from build123d import *

# Parameters (mm, degrees)
SKETCH1_W                 = 62.1
SKETCH1_H                 = 0.7
BASE_FLANGE1_DEPTH        = 87.8
EDGE_FLANGE1_DEPTH        = 87.8
EDGE_FLANGE2_DEPTH        = 87.8
EDGE_FLANGE3_DEPTH        = 62.1
CUT_EXTRUDE2_DEPTH        = 0.7
SKETCH14_R                = 1.7
CUT_EXTRUDE3_DEPTH        = 0.7
EDGE_FLANGE4_DEPTH        = 19
EDGE_FLANGE5_DEPTH        = 19
EDGE_FLANGE6_DEPTH        = 62.1
EDGE_FLANGE7_DEPTH        = 19
EDGE_FLANGE8_DEPTH        = 19
SKETCH32_W                = 10.5
SKETCH32_H                = 8
CUT_EXTRUDE5_DEPTH        = 0.7
FLAT_PATTERN1_START       = -20.7
FLAT_PATTERN1_OUTLINE_R   = 1.7
FLAT_PATTERN1_DEPTH       = 20
FLAT_PATTERN1_START_2     = -0.7
FLAT_PATTERN1_2_OUTLINE_R = 1.7
FLAT_PATTERN1_2_DEPTH     = 0.7


with BuildPart() as part:
    # Base-Flange1: sheet metal written as solids
    # Sketch1 → Base-Flange1 (new body)
    with BuildSketch(Plane.XY):
        with Locations((31.05, -0.35)):
            Rectangle(SKETCH1_W, SKETCH1_H)
    extrude(amount=BASE_FLANGE1_DEPTH)

    # Edge-Flange1: sheet metal written as solids
    # Edge-Flange1 section (on a plane across the edge) → Edge-Flange1 (add)
    with BuildSketch(Plane(origin=(63.1, -0.7, 0), x_dir=(-1, 0, 0), z_dir=(0, 0, 1))):
        with BuildLine():
            Line((-0.7, 1), (-0.7, 20))
            Line((-0.7, 20), (0, 20))
            Line((0, 20), (0, 1))
            ThreePointArc((0, 1), (0.292893219, 0.292893219), (1, 0))
            Line((1, 0), (1, -0.7))
            ThreePointArc((1, -0.7), (-0.202081528, -0.202081528), (-0.7, 1))
        make_face()
    extrude(amount=EDGE_FLANGE1_DEPTH)

    # Edge-Flange2: sheet metal written as solids
    # Edge-Flange2 section (on a plane across the edge) → Edge-Flange2 (add)
    with BuildSketch(Plane(origin=(-1, -0.7, 87.8), x_dir=(1, 0, 0), z_dir=(0, 0, -1))):
        with BuildLine():
            Line((-0.7, 1), (-0.7, 20))
            Line((-0.7, 20), (0, 20))
            Line((0, 20), (0, 1))
            ThreePointArc((0, 1), (0.292893219, 0.292893219), (1, 0))
            Line((1, 0), (1, -0.7))
            ThreePointArc((1, -0.7), (-0.202081528, -0.202081528), (-0.7, 1))
        make_face()
    extrude(amount=EDGE_FLANGE2_DEPTH)

    # Edge-Flange3: sheet metal written as solids
    # Edge-Flange3 section (on a plane across the edge) → Edge-Flange3 (add)
    with BuildSketch(Plane(origin=(62.1, -0.7, 88.8), x_dir=(0, 0, -1), z_dir=(-1, 0, 0))):
        with BuildLine():
            Line((-0.7, 1), (-0.7, 20))
            Line((-0.7, 20), (0, 20))
            Line((0, 20), (0, 1))
            ThreePointArc((0, 1), (0.292893219, 0.292893219), (1, 0))
            Line((1, 0), (1, -0.7))
            ThreePointArc((1, -0.7), (-0.202081528, -0.202081528), (-0.7, 1))
        make_face()
    extrude(amount=EDGE_FLANGE3_DEPTH)

    # Sketch13 → Cut-Extrude2 (cut)
    with BuildSketch(Plane.XY.offset(89.5)):
        with BuildLine():
            Line((38.05, -13.35), (38.05, -20.7))
            Line((38.05, -20.7), (48.05, -20.7))
            Line((48.05, -20.7), (48.05, -13.35))
            ThreePointArc((48.05, -13.35), (43.05, -8.35), (38.05, -13.35))
        make_face()
    extrude(amount=-CUT_EXTRUDE2_DEPTH, mode=Mode.SUBTRACT)

    # Sketch14 → Cut-Extrude3 (cut)
    with BuildSketch(Plane(origin=(0, 0, 0), x_dir=(1, 0, 0), z_dir=(0, 1, 0))):
        with Locations(Location((6.55, -7.2, 0), (0, 0, 270))):
            Circle(SKETCH14_R)
        with Locations(Location((55.55, -7.2, 0), (0, 0, 270))):
            Circle(SKETCH14_R)
        with Locations(Location((8.05, -80.7, 0), (0, 0, 270))):
            Circle(SKETCH14_R)
        with Locations(Location((54.05, -80.7, 0), (0, 0, 270))):
            Circle(SKETCH14_R)
    extrude(amount=-CUT_EXTRUDE3_DEPTH, mode=Mode.SUBTRACT)

    # Edge-Flange4: sheet metal written as solids
    # Edge-Flange4 section (on a plane across the edge) → Edge-Flange4 (add)
    with BuildSketch(Plane(origin=(64.1, -1.7, 88.8), x_dir=(-1, 0, 0), z_dir=(0, -1, 0))):
        with BuildLine():
            Line((-0.7, 2), (-0.7, 20))
            Line((-0.7, 20), (0, 20))
            Line((0, 20), (0, 2))
            ThreePointArc((0, 2), (0.585786438, 0.585786438), (2, 0))
            Line((2, 0), (2, -0.7))
            ThreePointArc((2, -0.7), (0.090811691, 0.090811691), (-0.7, 2))
        make_face()
    extrude(amount=EDGE_FLANGE4_DEPTH)

    # Edge-Flange5: sheet metal written as solids
    # Edge-Flange5 section (on a plane across the edge) → Edge-Flange5 (add)
    with BuildSketch(Plane(origin=(-2, -20.7, 88.8), x_dir=(1, 0, 0), z_dir=(0, 1, 0))):
        with BuildLine():
            Line((-0.7, 2), (-0.7, 20))
            Line((-0.7, 20), (0, 20))
            Line((0, 20), (0, 2))
            ThreePointArc((0, 2), (0.585786438, 0.585786438), (2, 0))
            Line((2, 0), (2, -0.7))
            ThreePointArc((2, -0.7), (0.090811691, 0.090811691), (-0.7, 2))
        make_face()
    extrude(amount=EDGE_FLANGE5_DEPTH)

    # Edge-Flange6: sheet metal written as solids
    # Edge-Flange6 section (on a plane across the edge) → Edge-Flange6 (add)
    with BuildSketch(Plane(origin=(0, -0.7, -1), x_dir=(0, 0, 1), z_dir=(1, 0, 0))):
        with BuildLine():
            Line((-0.7, 1), (-0.7, 20))
            Line((-0.7, 20), (0, 20))
            Line((0, 20), (0, 1))
            ThreePointArc((0, 1), (0.292893219, 0.292893219), (1, 0))
            Line((1, 0), (1, -0.7))
            ThreePointArc((1, -0.7), (-0.202081528, -0.202081528), (-0.7, 1))
        make_face()
    extrude(amount=EDGE_FLANGE6_DEPTH)

    # Edge-Flange7: sheet metal written as solids
    # Edge-Flange7 section (on a plane across the edge) → Edge-Flange7 (add)
    with BuildSketch(Plane(origin=(64.1, -20.7, -1), x_dir=(-1, 0, 0), z_dir=(0, 1, 0))):
        with BuildLine():
            Line((-0.7, 2), (-0.7, 20))
            Line((-0.7, 20), (0, 20))
            Line((0, 20), (0, 2))
            ThreePointArc((0, 2), (0.585786438, 0.585786438), (2, 0))
            Line((2, 0), (2, -0.7))
            ThreePointArc((2, -0.7), (0.090811691, 0.090811691), (-0.7, 2))
        make_face()
    extrude(amount=EDGE_FLANGE7_DEPTH)

    # Edge-Flange8: sheet metal written as solids
    # Edge-Flange8 section (on a plane across the edge) → Edge-Flange8 (add)
    with BuildSketch(Plane(origin=(-2, -1.7, -1), x_dir=(1, 0, 0), z_dir=(0, -1, 0))):
        with BuildLine():
            Line((-0.7, 2), (-0.7, 20))
            Line((-0.7, 20), (0, 20))
            Line((0, 20), (0, 2))
            ThreePointArc((0, 2), (0.585786438, 0.585786438), (2, 0))
            Line((2, 0), (2, -0.7))
            ThreePointArc((2, -0.7), (0.090811691, 0.090811691), (-0.7, 2))
        make_face()
    extrude(amount=EDGE_FLANGE8_DEPTH)

    # Sketch32 → Cut-Extrude5 (cut)
    with BuildSketch(Plane(origin=(0, 0, -1.7), x_dir=(-1, 0, 0), z_dir=(0, 0, -1))):
        with Locations((-49.8006007, -16.7)):
            Rectangle(SKETCH32_W, SKETCH32_H)
    extrude(amount=-CUT_EXTRUDE5_DEPTH, mode=Mode.SUBTRACT)

    # Flat-Pattern1: read off the stored shape, not the designer's step
    # Flat-Pattern1 outline → Flat-Pattern1 (cut)
    with BuildSketch(Plane(origin=(0, 0, 0), x_dir=(1, 0, 0), z_dir=(0, 1, 0)).offset(FLAT_PATTERN1_START)):
        with BuildLine():
            Line((-1.7, 0), (-1.7, -87.8))
            Line((-1.7, -87.8), (0, -87.8))
            Line((0, -87.8), (0, -88.5))
            Line((0, -88.5), (-1.053565375, -88.5))
            ThreePointArc((-1.053565375, -88.5), (-1.747445385, -87.772848716), (-2, -86.8))
            Line((-2, -86.8), (-2, -68.8))
            Line((-2, -68.8), (-2.7, -68.8))
            Line((-2.7, -68.8), (-2.7, -86.8))
            ThreePointArc((-2.7, -86.8), (-2.54495263, -87.701784958), (-2.097617696, -88.5))
            Line((-2.097617696, -88.5), (-18.7, -88.5))
            Line((-18.7, -88.5), (-18.7, -107.5))
            Line((-18.7, -107.5), (38.05, -107.5))
            Line((38.05, -107.5), (38.05, -100.15))
            ThreePointArc((38.05, -100.15), (43.05, -95.15), (48.05, -100.15))
            Line((48.05, -100.15), (48.05, -107.5))
            Line((48.05, -107.5), (80.8, -107.5))
            Line((80.8, -107.5), (80.8, -88.5))
            Line((80.8, -88.5), (64.197617696, -88.5))
            ThreePointArc((64.197617696, -88.5), (64.64495263, -87.701784958), (64.8, -86.8))
            Line((64.8, -86.8), (64.8, -68.8))
            Line((64.8, -68.8), (64.1, -68.8))
            Line((64.1, -68.8), (64.1, -86.8))
            ThreePointArc((64.1, -86.8), (63.847445385, -87.772848716), (63.153565375, -88.5))
            Line((63.153565375, -88.5), (62.1, -88.5))
            Line((62.1, -88.5), (62.1, -87.8))
            Line((62.1, -87.8), (63.8, -87.8))
            Line((63.8, -87.8), (63.8, 0))
            Line((63.8, 0), (62.1, 0))
            Line((62.1, 0), (62.1, 0.7))
            Line((62.1, 0.7), (63.153565375, 0.7))
            ThreePointArc((63.153565375, 0.7), (63.847445385, -0.027151284), (64.1, -1))
            Line((64.1, -1), (64.1, -19))
            Line((64.1, -19), (64.8, -19))
            Line((64.8, -19), (64.8, -1))
            ThreePointArc((64.8, -1), (64.009188309, 0.909188309), (62.1, 1.7))
            Line((62.1, 1.7), (0, 1.7))
            ThreePointArc((0, 1.7), (-1.909188309, 0.909188309), (-2.7, -1))
            Line((-2.7, -1), (-2.7, -19))
            Line((-2.7, -19), (-2, -19))
            Line((-2, -19), (-2, -1))
            ThreePointArc((-2, -1), (-1.747445385, -0.027151284), (-1.053565375, 0.7))
            Line((-1.053565375, 0.7), (0, 0.7))
            Line((0, 0.7), (0, 0))
            Line((0, 0), (-1.7, 0))
        make_face()
        with Locations((55.55, -7.2)):
            Circle(FLAT_PATTERN1_OUTLINE_R, mode=Mode.SUBTRACT)
        with Locations((8.05, -80.7)):
            Circle(FLAT_PATTERN1_OUTLINE_R, mode=Mode.SUBTRACT)
        with Locations((54.05, -80.7)):
            Circle(FLAT_PATTERN1_OUTLINE_R, mode=Mode.SUBTRACT)
        with Locations((6.55, -7.2)):
            Circle(FLAT_PATTERN1_OUTLINE_R, mode=Mode.SUBTRACT)
    extrude(amount=FLAT_PATTERN1_DEPTH, mode=Mode.SUBTRACT)

    # Flat-Pattern1 2 outline → Flat-Pattern1 2 (add)
    with BuildSketch(Plane(origin=(0, 0, 0), x_dir=(1, 0, 0), z_dir=(0, 1, 0)).offset(FLAT_PATTERN1_START_2)):
        with BuildLine():
            Line((0, -87.8), (0, -88.5))
            Line((0, -88.5), (-18.7, -88.5))
            Line((-18.7, -88.5), (-18.7, -107.5))
            Line((-18.7, -107.5), (38.05, -107.5))
            Line((38.05, -107.5), (38.05, -100.15))
            ThreePointArc((38.05, -100.15), (43.05, -95.15), (48.05, -100.15))
            Line((48.05, -100.15), (48.05, -107.5))
            Line((48.05, -107.5), (80.8, -107.5))
            Line((80.8, -107.5), (80.8, -88.5))
            Line((80.8, -88.5), (62.1, -88.5))
            Line((62.1, -88.5), (62.1, -87.8))
            Line((62.1, -87.8), (81.8, -87.8))
            Line((81.8, -87.8), (81.8, 0))
            Line((81.8, 0), (62.1, 0))
            Line((62.1, 0), (62.1, 0.7))
            Line((62.1, 0.7), (80.8, 0.7))
            Line((80.8, 0.7), (80.8, 19.7))
            Line((80.8, 19.7), (55.0506007, 19.7))
            Line((55.0506007, 19.7), (55.0506007, 11.7))
            Line((55.0506007, 11.7), (44.5506007, 11.7))
            Line((44.5506007, 11.7), (44.5506007, 19.7))
            Line((44.5506007, 19.7), (-18.7, 19.7))
            Line((-18.7, 19.7), (-18.7, 0.7))
            Line((-18.7, 0.7), (0, 0.7))
            Line((0, 0.7), (0, 0))
            Line((0, 0), (-19.7, 0))
            Line((-19.7, 0), (-19.7, -87.8))
            Line((-19.7, -87.8), (0, -87.8))
        make_face()
        with Locations((55.55, -7.2)):
            Circle(FLAT_PATTERN1_2_OUTLINE_R, mode=Mode.SUBTRACT)
        with Locations((8.05, -80.7)):
            Circle(FLAT_PATTERN1_2_OUTLINE_R, mode=Mode.SUBTRACT)
        with Locations((54.05, -80.7)):
            Circle(FLAT_PATTERN1_2_OUTLINE_R, mode=Mode.SUBTRACT)
        with Locations((6.55, -7.2)):
            Circle(FLAT_PATTERN1_2_OUTLINE_R, mode=Mode.SUBTRACT)
    extrude(amount=FLAT_PATTERN1_2_DEPTH)


solid = part.part
Build history of the part. All positions in model axes, mm. Give positions to 0.01 mm unless a question says otherwise; leave off trailing zeros. Loops run counter-clockwise (first coordinate to the right, second up) from the corner with the lowest first, then second, coordinate; pieces in that order, holes last. Notation, with made-up numbers: (53, -21.5) -> (74, -21.5) arc R18 cw to (74, -4.5) -> close; hole circle Ø3 at (-17, 61.25). An arc over 180 degrees is marked (long way). Answer in a Markdown table with one row per item.
Item 1: Slice it at A-A on z = 80.7. Write the cut outline in (x, y), plus the area to 3 significant figures.
Findings below:
| item | result |
|---|---|
| outline | (-19.7, -0.7) -> (6.35, -0.7) -> (6.35, 0) -> (-19.7, 0) -> close; (9.75, -0.7) -> (52.35, -0.7) -> (52.35, 0) -> (9.75, 0) -> close; (55.75, -0.7) -> (81.8, -0.7) -> (81.8, 0) -> (55.75, 0) -> close |
| area | 66.3 mm² |
Item 2: Mould opens along Z. For faces 1 (the cylindrical face through (42.94, -0.35, 95.15)), 2 (the flat face through (30, 0, 43)), 3 (the cylindrical face through (8.56, -0.35, 82.32)) say: pulls with the +Z half, pulls with the -Z half, needs draft (parallel to the pull), parting line crosses it, or undercut.
Findings below:
| item | result |
|---|---|
| face 1 | pulls with the +Z half |
| face 2 | needs draft |
| face 3 | undercut |
Item 3: Slice it at B-B on y = -0.4. Give the number of separate pieces and of enclosed holes in the cut face, plus the area to 3 significant figures.
Findings below:
| item | result |
|---|---|
| separate pieces | 1 |
| enclosed holes | 4 |
| area | 12,500 mm² |
Item 4: Flat gauge pins, fed straight in: P1, Ø4, axis at x = 17.5, z = 30.5, coming from the +Y side; P2, Ø2, axis at x = 8.05, z = 80.7, coming from the -Y side. Where does each tip first touch, or does it go through?
Findings below:
| item | result |
|---|---|
| P1 | stops at y = 0 |
| P2 | passes through |
Item 5: Probe line 1 along X through (y, z) = (-0.45, 80.7); line 2 along Z through (x, y) = (78, -0.5); line 3 along X through (y, z) = (-0.3, 7.2). List the from-to ranges inside material, lowest first. Write a range as [from, to].
Findings below:
| item | result |
|---|---|
| line 1 | x = [-19.7, 6.35], [9.75, 52.35], [55.75, 81.8] |
| line 2 | z = [-19.7, -0.7], [0, 87.8], [88.5, 107.5] |
| line 3 | x = [-19.7, 4.85], [8.25, 53.85], [57.25, 81.8] |
Item 6: Slice it at C-C on x = 50. Write the cut outline in (y, z).
Findings below:
| item | result |
|---|---|
| outline | (-0.7, -11.7) -> (0, -11.7) -> (0, 107.5) -> (-0.7, 107.5) -> close |
